```python
from build123d import *

# Parameters (mm, degrees)
F1_DEPTH      = 252.4125
F2_W          = 12.7
F2_H          = 6.35
F3_DEPTH      = 9.526
F3_DEPTH_BACK = 9.526


with BuildPart() as f1:
    # F0 (on Front) → F1 (new body, symmetric)
    with BuildSketch(Plane.XZ):
        Polygon((9.525, 7.9375), (-9.525, 7.9375), (-9.525, -7.9375), (9.525, -7.9375), (9.525, -3.175), (3.175, -3.175), (3.175, 3.175), (9.525, 3.175), align=None)
    extrude(amount=F1_DEPTH, both=True)

    # F2 (on Right) → F3 (cut, two sides)
    with BuildSketch(Plane.YZ) as f3_sk:
        with Locations((-246.0625, 0)):
            Rectangle(F2_W, F2_H)
        with Locations((246.0625, 0)):
            Rectangle(F2_W, F2_H)
    extrude(amount=-F3_DEPTH, mode=Mode.SUBTRACT)
    extrude(f3_sk.sketch, amount=F3_DEPTH_BACK, mode=Mode.SUBTRACT)


solid = f1.part
```
Work out the finished part from the listing and answer in its coordinate system (mm). Give positions to 0.01 mm unless a question says otherwise; leave off trailing zeros. Loops run counter-clockwise (first coordinate to the right, second up) from the corner with the lowest first, then second, coordinate; pieces in that order, holes last. Notation, with made-up numbers: (77, 62) -> (125, 62) arc R34 cw to (125, 98) -> close; hole circle Ø2 at (-3, -31.5). An arc over 180 degrees is marked (long way). Write item = value, one per line. Start each with the question number.
(1) The mould has two halves that part along Z. Classify faces 1 (the flat face through (0, -4, 7.938)), 2 (the flat face through (5, -1, -3.175)), 3 (the flat face through (0, -4, -7.938)): +Z half, -Z half, draft (parallel to the pull), parting line (faces both ways), or undercut.
(2) Find the intervals of material crossed by probe 1 along Z at (x, y) = (7.25, 62) (1 decimal); probe 2 along X at (y, z) = (65.5, 3) (3 decimals); probe 3 along Y at (x, z) = (0.75, 1), in increasing order. Write a range as from..to.
(3) Find section B-B on y = 42. Give the vertices of the cut face in (x, z) (1 decimal), and give its area (3 significant figures).
(4) Find section A-A on x = 6.5. Give the vertices of the cut face in (y, z) (1 decimal).
(5) Given pin 1 Ø3 at (y, z) = (-23.5, 0) entering from +X (3 decimals); pin 2 Ø7 at (x, z) = (-1, -0.5) entering from -Y; pin 3 Ø1.5 at (x, z) = (-2.5, -1.5) entering from +Y, each flat-ended and moving along its own axis, determine where each tip first touches the part or whether it passes through.
From the geometry:
q1.face_1 = +Z half
q1.face_2 = undercut
q1.face_3 = -Z half
q2.probe_1 = -7.9..-3.2, 3.2..7.9
q2.probe_2 = -9.525..3.175
q2.probe_3 = -239.71..239.71
q3.outline = (-9.5, -7.9) -> (9.5, -7.9) -> (9.5, -3.2) -> (3.2, -3.2) -> (3.2, 3.2) -> (9.5, 3.2) -> (9.5, 7.9) -> (-9.5, 7.9) -> close
q3.area = 262 mm^2
q4.outline = (-252.4, -7.9) -> (252.4, -7.9) -> (252.4, -3.2) -> (-252.4, -3.2) -> close; (-252.4, 3.2) -> (252.4, 3.2) -> (252.4, 7.9) -> (-252.4, 7.9) -> close
q5.pin_1 = 3.175
q5.pin_2 = -252.41
q5.pin_3 = 239.71
